```python
from build123d import *

# Parameters (mm, degrees)
F0_R     = 1.6
F1_DEPTH = 12.7


with BuildPart() as f1:
    # F0 (on Top) → F1 (new body)
    with BuildSketch(Plane.XY):
        with BuildLine():
            ThreePointArc((21, 16), (19.535534, 19.535534), (16, 21))
            Line((16, 21), (-16, 21))
            ThreePointArc((-16, 21), (-19.535534, 19.535534), (-21, 16))
            Line((-21, 16), (-21, -13.278688))
            Line((-21, -13.278688), (-12.540984, -21))
            Line((-12.540984, -21), (16, -21))
            ThreePointArc((16, -21), (19.535534, -19.535534), (21, -16))
            Line((21, -16), (21, 16))
        make_face()
        with BuildLine():
            ThreePointArc((-11.1, -17.6), (-12.7, -16), (-11.1, -14.4))
            Line((-11.1, -14.4), (-7.9, -14.4))
            ThreePointArc((-7.9, -14.4), (-6.3, -16), (-7.9, -17.6))
            Line((-7.9, -17.6), (-11.1, -17.6))
        make_face(mode=Mode.SUBTRACT)
        with Locations((16, -16)):
            Circle(F0_R, mode=Mode.SUBTRACT)
        with Locations((-16, 16)):
            Circle(F0_R, mode=Mode.SUBTRACT)
    extrude(amount=F1_DEPTH)


solid = f1.part
```
Design review of the part built by this model. Coordinates are the model's own, in mm. A direction names the side the tool comes from. Give positions to 0.01 mm unless a question says otherwise; leave off trailing zeros. Order: outer loops, then holes, each group sorted by start corner. A loop starts at its lowest first (then second) coordinate and runs counter-clockwise, first axis right, second up. Notation, with made-up numbers: (-27.75, 0) - (26.25, 0) arc R31 ccw to (26.25, 31) - close; hole circle Ø8 at (37, 4). An arc over 180 degrees is marked (long way). Use a Markdown table: item, result. Add a question column.
(1) Clearance check with a flat-ended pin moving along its axis: P1, Ø4, axis at x = -16, y = 16, coming from the +Z side. State where the tip first meets the part, or that it passes through.
(2) Wall thickness on probe 1 along Y at (x, z) = (-8, 10.75); probe 2 along Y at (x, z) = (-16, 7.25); probe 3 along Y at (x, z) = (-18, 1.75): over which ranges is each line inside the solid? List them lowest first. Write a range as [from, to].
(3) Machinability: for faces 1 (the face through (-21, 2, 6)), 2 (the face through (-9, -17.6, 6)), which of the approach directions +Z, -Z, +X, -X, +Y, -Y give a long, thin tool a straight path to every point of the face, cutting with its end or side? Answer none if there is none.
(4) Add section A-A on z = 11.5. Give the boundary of the cut face in (x, y).
(5) Mouldability with a two-part tool opening along X and no side actions: class faces 3 (the face through (-16.83, -17.085, 6.261)), 4 (the face through (21, 0, 6)), 5 (the face through (-17.18, 17.08, 6.26)) as +X half, -X half, draft (parallel to the pull), parting line (faces both ways), or undercut.
Report:
| question | item | result |
|---|---|---|
| 1 | P1 | stops at z = 12.7 |
| 2 | probe 1 | y = [-21, -17.6], [-14.4, 21] |
| 2 | probe 2 | y = [-17.84, 14.4], [17.6, 21] |
| 2 | probe 3 | y = [-16.02, 20.58] |
| 3 | face 1 | +Z, -Z, -X, +Y, -Y |
| 3 | face 2 | +Z, -Z |
| 4 | outline | (-21, -13.28) - (-12.54, -21) - (16, -21) arc R5 ccw to (21, -16) - (21, 16) arc R5 ccw to (16, 21) - (-16, 21) arc R5 ccw to (-21, 16) - close; hole circle Ø3.2 at (-16, 16); hole (-11.1, -17.6) - (-7.9, -17.6) arc R1.6 ccw to (-7.9, -14.4) - (-11.1, -14.4) arc R1.6 ccw to start; hole circle Ø3.2 at (16, -16) |
| 5 | face 3 | -X half |
| 5 | face 4 | +X half |
| 5 | face 5 | undercut |
